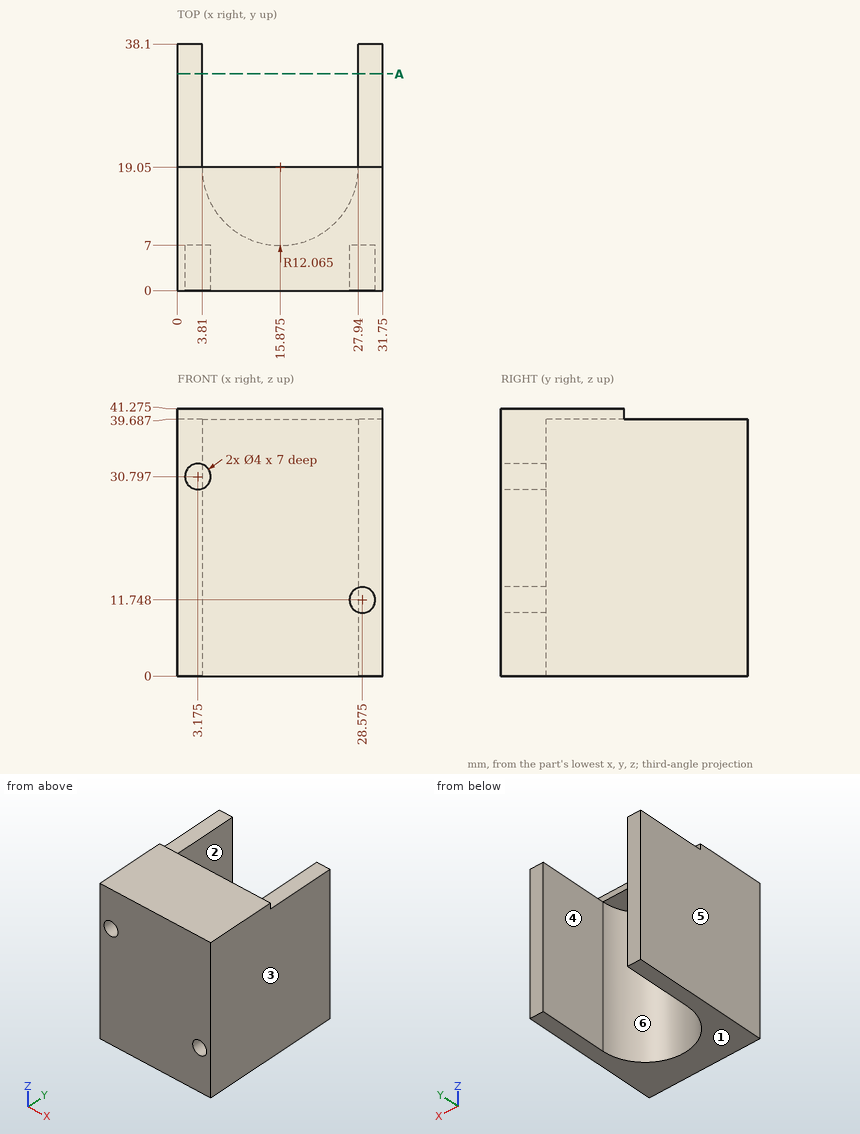
Input: dimensioned drawing with shaded views. Units: mm. Origin: part minimum x, y, z. A direction names the side the tool comes from. Coordinates: 2 decimals unless noted, no trailing zeros. Order: outer loops, then holes, each group sorted by start corner. A loop starts at its lowest first (then second) coordinate and runs counter-clockwise, first axis right, second up. Notation, with made-up numbers: (9.25, 78) - (31.25, 78) arc R14 ccw to (31.25, 87) - close; hole circle Ø5 at (73, 53.5). An arc over 180 degrees is marked (long way). Put each result on its own line as item: value.
1. Draft query along X for the marked faces 1, 2 and 3. Return one class per face: pulls with the +X half, pulls with the -X half, needs draft (parallel to the pull), parting line crosses it, or undercut.
Report:
face 1: needs draft
face 2: undercut
face 3: pulls with the +X half
2. Line query: line 1 along X through (y, z) = (25.5, 39); line 2 along Z through (x, y) = (10, 19) (1 decimal); line 3 along X through (y, z) = (13.5, 9). Output: solid intervals per line, ascending.
Report:
line 1: x = 0 to 3.81, 27.94 to 31.75
line 2: z = 39.7 to 41.3
line 3: x = 0 to 5.16, 26.59 to 31.75
3. Contact query for flat-ended pins moving along their axis: pin 1 Ø1.1 at (x, y) = (30, 28) entering from +Z; pin 2 Ø1.3 at (x, z) = (22, 40.5) entering from +Y; pin 3 Ø2 at (x, z) = (3.5, 31) entering from -Y. Output: stop coordinate, or through.
Report:
pin 1: stops at z = 39.69
pin 2: stops at y = 19.05
pin 3: stops at y = 7
4. Reachability of the marked faces 4, 5 and 6 from +Z, -Z, +X, -X, +Y, -Y: full face, straight path, thin tool, end or side. Return the list, or none.
Report:
face 4: +Z, -Z, +Y
face 5: +Z, -Z, -X, +Y, -Y
face 6: -Z, +Y
5. Cut plane A-A on y = 33.5. Return the cut outline in (x, z).
Report:
outline: (0, 0) - (3.81, 0) - (3.81, 39.69) - (0, 39.69) - close; (27.94, 0) - (31.75, 0) - (31.75, 39.69) - (27.94, 39.69) - close
